from build123d import *

# Parameters (mm, degrees)
SKETCH2_R             = 5
SKETCH4_R             = 5
BOSS_EXTRUDE1_DEPTH   = 55
CRVPATTERN1_START     = -1e-07
CRVPATTERN1_OUTLINE_R = 5
CRVPATTERN1_DEPTH     = 55.0000001


# Read off the part's stored shape, not the designer's step: CrvPattern1
with BuildPart() as part:
    # Sweep1: sweep along a path in Sketch1
    with BuildLine(Plane.XY) as sweep1_path:
        Line((0, 197.5), (62.586692935, 197.5))
        ThreePointArc((62.586692935, 197.5), (68.542028244, 195.533304511), (72.154897335, 190.406796273))
        Line((72.154897335, 190.406796273), (130, 0))
    # Sketch2 → Sweep1 (sweep)
    with BuildSketch(Plane(origin=(0, 0, 0), x_dir=(0, 0, -1), z_dir=(1, 0, 0))):
        with Locations((0, 197.5)):
            Circle(SKETCH2_R)
    sweep1 = sweep(path=sweep1_path.line)

    # Sketch4 → Boss-Extrude1 (add)
    with BuildSketch(Plane.XY):
        with Locations(Location((126.387902166, 11.889822036, 0), (0, 0, 196.898648694))):
            Circle(SKETCH4_R)
    extrude(amount=BOSS_EXTRUDE1_DEPTH)

    # CrvPattern1 outline → CrvPattern1 (add)
    with BuildSketch(Plane.XY.offset(CRVPATTERN1_START)):
        with Locations((119.120911483, 35.810333034)):
            Circle(CRVPATTERN1_OUTLINE_R)
        with Locations((111.8539208, 59.730844032)):
            Circle(CRVPATTERN1_OUTLINE_R)
        with Locations((104.586930117, 83.65135503)):
            Circle(CRVPATTERN1_OUTLINE_R)
        with Locations((97.319939434, 107.571866029)):
            Circle(CRVPATTERN1_OUTLINE_R)
        with Locations((90.052948751, 131.492377027)):
            Circle(CRVPATTERN1_OUTLINE_R)
        with Locations((82.785958068, 155.412888025)):
            Circle(CRVPATTERN1_OUTLINE_R)
        with Locations((75.518967385, 179.333399023)):
            Circle(CRVPATTERN1_OUTLINE_R)
        with Locations((61.918405072, 197.5)):
            Circle(CRVPATTERN1_OUTLINE_R)
        with Locations((36.918405072, 197.5)):
            Circle(CRVPATTERN1_OUTLINE_R)
    crvpattern1 = extrude(amount=CRVPATTERN1_DEPTH)

    # Mirror1: Sweep1, CrvPattern1 across plane
    add(sweep1.mirror(Plane.XY.offset(27.5)))
    add(crvpattern1.mirror(Plane.XY.offset(27.5)))


solid = part.part
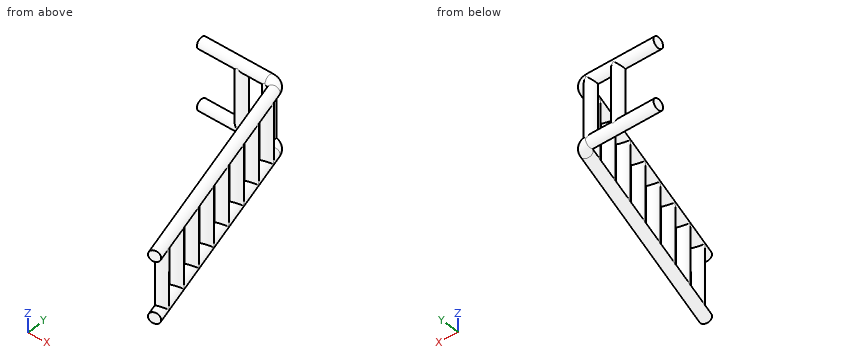
CAD build for the part. Positions are in the model's coordinates, mm. Coordinates: 2 decimals unless noted, no trailing zeros.
Item 1: Band-saw the part on A-A on z = 43. Give the number of separate pieces and of enclosed holes in the cut face, plus the area to 3 significant figures.
Check sheet entries:
separate pieces: 10
enclosed holes: 0
area: 785 mm2
Item 2: Drill centre lines: L1, parallel to Z at x = 82.5, y = 140.5; L2, parallel to Y at x = 97, z = 41; L3, parallel to Z at x = 126, y = 17. Where is each one in solid material? Low to high.
Check sheet entries:
L1: z = -1.94 to 1.94, 53.06 to 56.94
L2: y = 102.58 to 112.56
L3: z = -4.87 to 4.87, 50.13 to 59.87
Item 3: Pin check, flat tips, straight feed: pin 1 Ø8 at (y, z) = (120, 1.5) entering from -X; pin 2 Ø1.5 at (x, z) = (20, 52) entering from +Y; pin 3 Ø10 at (x, z) = (43, 13.5) entering from +Y. Stop position of each tip, or through.
Check sheet entries:
pin 1: stops at x = 87.17
pin 2: stops at y = 201.97
pin 3: stops at y = 202.38
